Verification items for the finished model (mm, model axes). Coordinates: 2 decimals unless noted, no trailing zeros. Loops run counter-clockwise (first coordinate to the right, second up) from the corner with the lowest first, then second, coordinate; pieces in that order, holes last. Notation, with made-up numbers: (81.25, 34) -> (135.25, 34) arc R21 ccw to (135.25, 47) -> close; hole circle Ø3 at (-28.75, 31.25). An arc over 180 degrees is marked (long way). Use CSV: the item, a comma, the result in double quotes. Start each with the question number.
```python
from build123d import *

# Parameters (mm, degrees)
SKETCH1_W           = 58
SKETCH1_H           = 58
SKETCH1_R           = 20
SKETCH1_R_2         = 2.5
BOSS_EXTRUDE1_DEPTH = 3


with BuildPart() as part:
    # Sketch1 → Boss-Extrude1 (new body)
    with BuildSketch(Plane(origin=(0, 0, 0), x_dir=(1, 0, 0), z_dir=(0, 1, 0))):
        with Locations((29, -29)):
            Rectangle(SKETCH1_W, SKETCH1_H)
        with Locations((29, -29)):
            Circle(SKETCH1_R, mode=Mode.SUBTRACT)
        with Locations((5.5, -5.5)):
            Circle(SKETCH1_R_2, mode=Mode.SUBTRACT)
        with Locations((52.5, -5.5)):
            Circle(SKETCH1_R_2, mode=Mode.SUBTRACT)
        with Locations((52.5, -52.5)):
            Circle(SKETCH1_R_2, mode=Mode.SUBTRACT)
        with Locations((5.5, -52.5)):
            Circle(SKETCH1_R_2, mode=Mode.SUBTRACT)
    extrude(amount=BOSS_EXTRUDE1_DEPTH)


solid = part.part
```
1. Release check for a two-part mould opening along X. For faces 1 (the cylindrical face through (54.81, 1.48, 6.46)), 2 (the flat face through (29, 1, 58)), 3 (the flat face through (0, 1, 29)) record: released by +X, released by -X, zero draft, split by the parting line, or undercut.
2. Cross-section at B-B, the plane x = 41. Record the boundary of the cut face in (y, z), plus the area to 3 significant figures.
3. Cross-section at A-A, the plane z = 5.5. Record the boundary of the cut face in (x, y), plus the area to 3 significant figures.
4. Cross-section at D-D, the plane z = 36. Record the boundary of the cut face in (x, y) (3 decimals), plus the area to 3 significant figures.
5. Scan lines: line 1 (Z direction, x = 52.5, y = 2); line 2 (X direction, y = 2.15, z = 29). Record each from-to range of solid material in increasing order.
6. Cross-section at C-C, the plane y = 2.45. Record the boundary of the cut face in (x, z), plus the area to 3 significant figures.
Solution:
1,face 1,"undercut"
1,face 2,"zero draft"
1,face 3,"released by -X"
2,outline,"(0, 0) -> (3, 0) -> (3, 13) -> (0, 13) -> close; (0, 45) -> (3, 45) -> (3, 58) -> (0, 58) -> close"
2,area,"78.0 mm2"
3,outline,"(0, 0) -> (3, 0) -> (3, 3) -> (0, 3) -> close; (8, 0) -> (50, 0) -> (50, 3) -> (8, 3) -> close; (55, 0) -> (58, 0) -> (58, 3) -> (55, 3) -> close"
3,area,"144 mm2"
4,outline,"(0, 0) -> (10.265, 0) -> (10.265, 3) -> (0, 3) -> close; (47.735, 0) -> (58, 0) -> (58, 3) -> (47.735, 3) -> close"
4,area,"61.6 mm2"
5,line 1,"z = 0 to 3, 8 to 50, 55 to 58"
5,line 2,"x = 0 to 9, 49 to 58"
6,outline,"(0, 0) -> (58, 0) -> (58, 58) -> (0, 58) -> close; hole circle Ø5 at (5.5, 5.5); hole circle Ø5 at (5.5, 52.5); hole circle Ø40 at (29, 29); hole circle Ø5 at (52.5, 5.5); hole circle Ø5 at (52.5, 52.5)"
6,area,"2,030 mm2"
